from build123d import *

# Parameters (mm, degrees)
SKETCH2_W           = 179.5
SKETCH2_H           = 179.5
BOSS_EXTRUDE1_DEPTH = 5
BOSS_EXTRUDE2_DEPTH = 60
SKETCH4_W           = 20
SKETCH4_H           = 40.8
SKETCH4_R           = 2.25
CUT_EXTRUDE1_DEPTH  = 5
CUT_EXTRUDE2_START  = -5
CUT_EXTRUDE2_DEPTH  = 50.8
SKETCH6_R           = 1.1
CUT_EXTRUDE3_DEPTH  = 5
SKETCH7_W           = 5
SKETCH7_H           = 50
BOSS_EXTRUDE3_DEPTH = 60


with BuildPart() as part:
    # Sketch2 → Boss-Extrude1 (new body)
    with BuildSketch(Plane(origin=(0, 0, 0), x_dir=(1, 0, 0), z_dir=(0, 1, 0))):
        Rectangle(SKETCH2_W, SKETCH2_H)
    extrude(amount=BOSS_EXTRUDE1_DEPTH)

    # Sketch3 → Boss-Extrude2 (add)
    with BuildSketch(Plane(origin=(0, 5, 0), x_dir=(1, 0, 0), z_dir=(0, 1, 0))):
        with BuildLine():
            Line((-14.325373702, 26.15370755), (-11.374207646, 29.984724331))
            Line((-11.374207646, 29.984724331), (-18.474207646, 42.282285065))
            Line((-18.474207646, 42.282285065), (-18.474207646, 47.217714935))
            Line((-18.474207646, 47.217714935), (-11.374207646, 59.515275669))
            Line((-11.374207646, 59.515275669), (-14.325373702, 63.34629245))
            ThreePointArc((-14.325373702, 63.34629245), (-23.474207646, 44.75), (-14.325373702, 26.15370755))
        make_face()
        with BuildLine():
            Line((11.374207646, 29.984724331), (14.325373702, 26.15370755))
            ThreePointArc((14.325373702, 26.15370755), (21.063181402, 34.387528584), (23.474207646, 44.75))
            ThreePointArc((23.474207646, 44.75), (21.063181402, 55.112471416), (14.325373702, 63.34629245))
            Line((14.325373702, 63.34629245), (11.374207646, 59.515275669))
            Line((11.374207646, 59.515275669), (18.474207646, 47.217714935))
            Line((18.474207646, 47.217714935), (18.474207646, 42.282285065))
            Line((18.474207646, 42.282285065), (11.374207646, 29.984724331))
        make_face()
        with BuildLine():
            Line((-7.1, 27.517009396), (-11.374207646, 29.984724331))
            Line((-11.374207646, 29.984724331), (-14.325373702, 26.15370755))
            ThreePointArc((-14.325373702, 26.15370755), (0, 21.275792354), (14.325373702, 26.15370755))
            Line((14.325373702, 26.15370755), (11.374207646, 29.984724331))
            Line((11.374207646, 29.984724331), (7.1, 27.517009396))
            Line((7.1, 27.517009396), (-7.1, 27.517009396))
        make_face()
    extrude(amount=BOSS_EXTRUDE2_DEPTH)

    # Sketch4 → Cut-Extrude1 (cut)
    with BuildSketch(Plane(origin=(0, 5, 0), x_dir=(1, 0, 0), z_dir=(0, 1, 0))):
        with Locations((0, -10.65)):
            Rectangle(SKETCH4_W, SKETCH4_H)
        with Locations((0, -0.25)):
            Circle(SKETCH4_R, mode=Mode.SUBTRACT)
        with Locations((0, -0.25)):
            Circle(SKETCH4_R)
    extrude(amount=-CUT_EXTRUDE1_DEPTH, mode=Mode.SUBTRACT)

    # Sketch5 → Cut-Extrude2 (cut)
    with BuildSketch(Plane.XY.offset(-9.75).offset(CUT_EXTRUDE2_START)):
        with BuildLine():
            Line((-1, 5), (-0.735509529, 3.5))
            ThreePointArc((-0.735509529, 3.5), (0, 3.177514378), (0.735509529, 3.5))
            Line((0.735509529, 3.5), (1, 5))
            Line((1, 5), (-1, 5))
        make_face()
    extrude(amount=CUT_EXTRUDE2_DEPTH, mode=Mode.SUBTRACT)

    # Sketch6 → Cut-Extrude3 (cut)
    with BuildSketch(Plane(origin=(0, 5, 0), x_dir=(1, 0, 0), z_dir=(0, 1, 0))):
        with Locations(Location((-5, 14.5, 0), (0, 0, 270))):
            Circle(SKETCH6_R)
        with Locations(Location((5, 14.5, 0), (0, 0, 270))):
            Circle(SKETCH6_R)
        with Locations(Location((5, -35.8, 0), (0, 0, 270))):
            Circle(SKETCH6_R)
        with Locations(Location((-5, -35.8, 0), (0, 0, 270))):
            Circle(SKETCH6_R)
    extrude(amount=-CUT_EXTRUDE3_DEPTH, mode=Mode.SUBTRACT)

    # Sketch7 → Boss-Extrude3 (add)
    with BuildSketch(Plane(origin=(0, 5, 0), x_dir=(1, 0, 0), z_dir=(0, 1, 0))):
        with Locations((-40.25, -64.75)):
            Rectangle(SKETCH7_W, SKETCH7_H)
        Polygon((-89.75, -34.75), (-89.75, -39.75), (-42.75, -39.75), (-37.75, -39.75), (-37.75, -34.75), align=None)
    extrude(amount=BOSS_EXTRUDE3_DEPTH)


solid = part.part
CAD build for the part. Positions are in the model's coordinates, mm. A direction names the side the tool comes from. Round coordinates to 2 decimals unless told otherwise and drop trailing zeros. Write each loop counter-clockwise with the first axis right and the second up, starting at its lowest first coordinate (ties: lowest second). Pieces come first, ordered by that corner, then holes.
(1) 3-axis set-ups, long thin cutter, end or side, ignore diameter. For faces 1 (the face through (0, 3, 31.05)), 2 (the face through (14.875, 34.58, -53.453)), 3 (the face through (-37.75, 35, 63)): which of +Z, -Z, +X, -X, +Y, -Y reach the whole face in a straight line?
(2) Mould opens along X. For faces 4 (the face through (-67, 35, 39.75)), 5 (the face through (18.474, 35, -45)), 6 (the face through (-89.75, 3, 0)), 7 (the face through (-14.875, 34.58, -36.047)) say: pulls with the +X half, pulls with the -X half, needs draft (parallel to the pull), parting line crosses it, or undercut.
(3) Slice it at B-B, the plane x = -72. Write the cut outline in (y, z), and give its area (3 significant figures).
(4) Probe line 1 along X through (y, z) = (2.75, -14.5); line 2 along X through (y, z) = (3.7, 35.8); line 3 along X through (y, z) = (1, -14). List the from-to ranges inside material, lowest first.
(5) Slice it at D-D, the plane z = 66.5. Write the cut outline in (x, y), and give its area (3 significant figures).
(6) Drop flat-ended pins along their axis: P1, Ø10, axis at x = -62.5, z = 53.5, coming from the +Y side; P2, Ø4, axis at y = 45.5, z = -45, coming from the +X side; P3, Ø5, axis at x = -46.5, y = 36.5, coming from the -Z side; P4, Ø10, axis at x = 71.5, y = 12.5, coming from the +Z side. Give the stop position or say it passes through.
(7) Slice it at A-A, the plane y = 7.5. Write the cut outline in (x, z).
(8) Slice it at C-C, the plane z = 10. Write the cut outline in (x, y), and give its area (4 significant figures).
From the geometry:
1. face 1: +Y, -Y
1. face 2: +Y
1. face 3: +Z, -Z, +X, +Y
2. face 4: needs draft
2. face 5: undercut
2. face 6: pulls with the -X half
2. face 7: undercut
3. outline: (0, -89.75) - (5, -89.75) - (5, 34.75) - (65, 34.75) - (65, 39.75) - (5, 39.75) - (5, 89.75) - (0, 89.75) - close
3. area: 1,200 mm2
4. line 1: x = -89.75 to -6.1, -3.9 to 3.9, 6.1 to 89.75
4. line 2: x = -89.75 to -6.1, -3.9 to -0.77, 0.77 to 3.9, 6.1 to 89.75
4. line 3: x = -89.75 to -5.98, -4.02 to 4.02, 5.98 to 89.75
5. outline: (-89.75, 0) - (89.75, 0) - (89.75, 5) - (-37.75, 5) - (-37.75, 65) - (-42.75, 65) - (-42.75, 5) - (-89.75, 5) - close
5. area: 1,200 mm2
6. P1: stops at y = 5
6. P2: stops at x = 23.47
6. P3: stops at z = 34.75
6. P4: passes through
7. outline: (-89.75, 34.75) - (-37.75, 34.75) - (-37.75, 89.75) - (-42.75, 89.75) - (-42.75, 39.75) - (-89.75, 39.75) - close; (-18.47, -47.22) - (-18.47, -42.28) - (-11.37, -29.98) - (-7.1, -27.52) - (7.1, -27.52) - (11.37, -29.98) - (18.47, -42.28) - (18.47, -47.22) - (11.37, -59.52) - (14.33, -63.35) arc R23.47 ccw (long way) to (-14.33, -63.35) - (-11.37, -59.52) - close
8. outline: (-89.75, 0) - (-10, 0) - (-10, 5) - (-89.75, 5) - close; (10, 0) - (89.75, 0) - (89.75, 5) - (10, 5) - close
8. area: 797.5 mm2
